The model under review builds one solid part; all positions refer to its coordinate system, in mm. Coordinates: 2 decimals unless noted, no trailing zeros. Write each loop counter-clockwise with the first axis right and the second up, starting at its lowest first coordinate (ties: lowest second). Pieces come first, ordered by that corner, then holes.
Autodesk Inventor part; units mm, degrees
ref_plane "YZ Plane" through (0, 0, 0) normal (1, 0, 0) x (0, 1, 0)
ref_plane "XZ Plane" through (0, 0, 0) normal (0, 1, 0) x (-1, 0, 0)
ref_plane "XY Plane" through (0, 0, 0) normal (0, 0, 1) x (1, 0, 0)
ref_plane "Work Plane1" through (0, 0, 0) normal (0, 0, 1) x (1, 0, 0)
sketch "Sketch1" plane through (0, 0, 0) normal (0, 0, 1) x (1, 0, 0)
  line L0 (0, 0) -> (-152.4, 0)
  circle A0 centre (-38.1, -165.1) radius 2.8067 construction
  line L1 (-60.3956, -177.0525) -> (-38.9279, -182.8048)
  line L2 (-127.7475, -244.4044) -> (-121.9952, -265.8721)
  arc A1 (-127.7475, -244.4044) -> (-60.3956, -177.0525) centre (-152.4, -152.4) ccw
  arc A2 (-121.9952, -265.8721) -> (-38.9279, -182.8048) centre (-152.4, -152.4) ccw
  line L3 (0, 0) -> (-63.5, 0)
  line L4 (-63.5, 0) -> (-63.5, -215.9) construction
  line L5 (-63.5, -215.9) -> (-88.9, -215.9) construction
  line L6 (-88.9, -215.9) -> (-88.9, -241.3) construction
  circle A3 centre (-63.5, -215.9) radius 3.302
  circle A4 centre (-88.9, -241.3) radius 3.302
  dimension "d0" = 152.4
  dimension "d8" = 63.5
  dimension "d9" = 215.9
  dimension "d10" = 25.4
  dimension "d11" = 25.4
  dimension "d12" = 6.604
  dimension "d13" = 6.604
extrude "Extrusion1" add sketch "Sketch1" along normal blind 6.35
properties part number "vrRig_v08_ballCupAlignment"
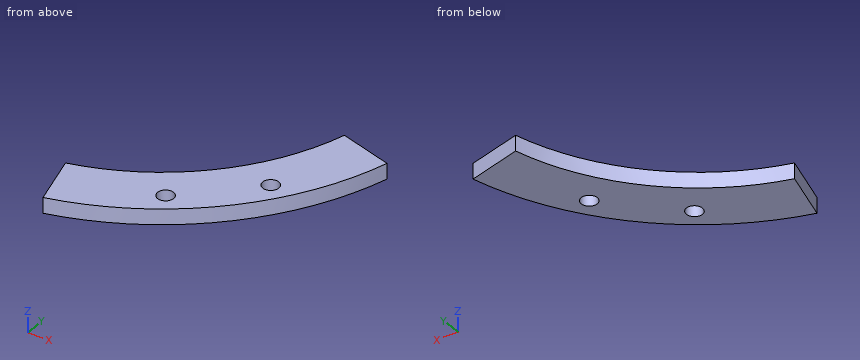
Item 1: Take a section at B-B, the plane y = -241.3. Write out the cut boundary in (x, z), plus the area to 3 significant figures.
Solved:
outline: (-118.2, 0) - (-92.2, 0) - (-92.2, 6.35) - (-118.2, 6.35) - close; (-85.6, 0) - (-75.61, 0) - (-75.61, 6.35) - (-85.6, 6.35) - close
area: 229 mm2
Item 2: Take a section at C-C, the plane z = 5. Write out the cut boundary in (x, y), plus the area to 3 significant figures.
Solved:
outline: (-127.75, -244.4) - (-122, -265.87) arc R117.47 ccw to (-38.93, -182.8) - (-60.4, -177.05) arc R95.25 cw to start; hole circle Ø6.6 at (-88.9, -241.3); hole circle Ø6.6 at (-63.5, -215.9)
area: 2,410 mm2
Item 3: For pin 1 (4 mm diameter, centred on x = -63.5, y = -215.9, fed in from -Z); pin 2 (1.5 mm diameter, centred on y = -197.5, z = 4.5, fed in from -X); pin 3 (3 mm diameter, centred on x = -91, z = 4.5, fed in from -Y), all flat-tipped, find the tip position at first contact; note any pin that passes through.
Solved:
pin 1: passes through
pin 2: stops at x = -68.91
pin 3: stops at y = -253.46
Item 4: Take a section at A-A, the plane x = -88.9. Write out the cut boundary in (y, z).
Solved:
outline: (-251.23, 0) - (-244.6, 0) - (-244.6, 6.35) - (-251.23, 6.35) - close; (-238, 0) - (-223.4, 0) - (-223.4, 6.35) - (-238, 6.35) - close
Item 5: To check wall thickness, follow line 1 along Y through (x, z) = (-88.9, 2); line 2 along Y through (x, z) = (-89, 4); line 3 along X through (y, z) = (-213, 5.5). State the ranges of each line that lie inside material, in increasing order.
Solved:
line 1: y = -251.23 to -244.6, -238 to -223.4
line 2: y = -251.3 to -244.6, -238 to -223.48
line 3: x = -78.91 to -65.08, -61.92 to -51.76
Item 6: Take a section at D-D, the plane x = -110. Write out the cut boundary in (y, z).
Solved:
outline: (-261.96, 0) - (-237.69, 0) - (-237.69, 6.35) - (-261.96, 6.35) - close
